Model file for the job. Use its own axes, mm. A direction names the side the tool comes from. Coordinates: 2 decimals unless noted, no trailing zeros. Write each loop counter-clockwise with the first axis right and the second up, starting at its lowest first coordinate (ties: lowest second). Pieces come first, ordered by that corner, then holes. Notation, with made-up numbers: M 25.5,64.5 L 82.5,64.5 A29 ccw 82.5,95.5 Z; hole C 82.5,85 d6. An arc over 180 degrees is marked long. Put each result on its own line as item: value. Start each with the question number.
Q1. Drop flat-ended pins along their axis: pin 1 (4 mm diameter, centred on x = -2, y = 6, fed in from +Z); pin 2 (2 mm diameter, centred on x = -15, z = 3, fed in from +Y). Give the stop position or say it passes through.
Q2. Cut at A-A (z = 8). Write the cut outline in (x, y), then the cut area to 3 significant figures.
Q3. Cut at C-C (x = -1.5). Write the cut outline in (y, z), then the cut area to 3 significant figures.
Q4. Which spindle directions (+Z, -Z, +X, -X, +Y, -Y) get a long thin tool onto all of the face, cutting with end or side? Do faces 4 (the flat face through (0, 0, 0)), 5 (the flat face through (0, 0, 1)). Say none if no direction does.
Q5. Cut at B-B (y = 3.5). Write the cut outline in (x, z), then the cut area to 3 significant figures.
Q6. Drill centre lines: line 1 along X through (y, z) = (23.5, 15.25); line 2 along Z through (x, y) = (0, -24); line 3 along X through (y, z) = (-12, 1.75). Where is each one in solid material? Low to high.
Q7. Pull direction X, two halves, no side cores. Call faces 1 (the cylindrical face through (-21.93, 0.44, 1.6)), 2 (the flat face through (-23.5, 0, 12)), 3 (the cylindrical face through (22.64, 0.44, 0.9)): pulls with the +X half, pulls with the -X half, needs draft (parallel to the pull), parting line crosses it, or undercut.
Q8. Cut at D-D (z = 2.25). Write the cut outline in (x, y), then the cut area to 3 significant figures.
```python
from build123d import *

# Parameters (mm, degrees)
F0_W     = 47
F0_H     = 62.5
F1_DEPTH = 21
F2_R     = 3
F3_T     = -1


with BuildPart() as f1:
    # F0 (on Top) → F1 (new body)
    with BuildSketch(Plane.XY):
        Rectangle(F0_W, F0_H)
    extrude(amount=F1_DEPTH)

    # F2
    f2_edges = [f1.edges().sort_by_distance(p)[0] for p in [
        (23.5, 0, 0),
        (-23.5, 0, 0),
    ]]
    fillet(f2_edges, radius=F2_R)

    # F3
    f3_openings = [f1.faces().sort_by_distance(p)[0] for p in [
        (0, 0, 21),
        (0, -31.25, 10.538623),
        (0, 31.25, 10.538623),
    ]]
    offset(amount=F3_T, openings=f3_openings)


solid = f1.part
```
Computed values:
1. pin 1: z = 1
1. pin 2: through
2. outline: M -23.5,-31.25 L -22.5,-31.25 L -22.5,31.25 L -23.5,31.25 Z; M 22.5,-31.25 L 23.5,-31.25 L 23.5,31.25 L 22.5,31.25 Z
2. area: 125 mm2
3. outline: M -31.25,0 L 31.25,0 L 31.25,1 L -31.25,1 Z
3. area: 62.5 mm2
4. face 4: -Z, +X, -X, +Y, -Y
4. face 5: +Z, +Y, -Y
5. outline: M -23.5,3 A3 ccw -20.5,0 L 20.5,0 A3 ccw 23.5,3 L 23.5,21 L 22.5,21 L 22.5,3 A2 cw 20.5,1 L -20.5,1 A2 cw -22.5,3 L -22.5,21 L -23.5,21 Z
5. area: 84.9 mm2
6. line 1: -23.5 to -22.5, 22.5 to 23.5
6. line 2: 0 to 1
6. line 3: -23.23 to -22.06, 22.06 to 23.23
7. face 1: undercut
7. face 2: pulls with the -X half
7. face 3: pulls with the +X half
8. outline: M -23.4,-31.25 L -22.35,-31.25 L -22.35,31.25 L -23.4,31.25 Z; M 22.35,-31.25 L 23.4,-31.25 L 23.4,31.25 L 22.35,31.25 Z
8. area: 131 mm2
